CAD build for the part. Positions are in the model's coordinates, mm. A direction names the side the tool comes from. Round coordinates to 2 decimals unless told otherwise and drop trailing zeros. Loops run counter-clockwise (first coordinate to the right, second up) from the corner with the lowest first, then second, coordinate; pieces in that order, holes last.
```python
from build123d import *

# Parameters (mm, degrees)
SKETCH1_W           = 24
SKETCH1_H           = 24
BOSS_EXTRUDE1_DEPTH = 20
SKETCH5_W           = 5
SKETCH5_H           = 4
SKETCH3_W           = 20
SKETCH3_H           = 20
CUT_EXTRUDE5_DEPTH  = 6
SKETCH14_W          = 20
SKETCH14_H          = 20
CUT_EXTRUDE6_DEPTH  = 2
SKETCH15_W          = 17.5
SKETCH15_H          = 17.5
CUT_EXTRUDE7_DEPTH  = 9
CUT_EXTRUDE8_REACH  = 5
SKETCH16_R          = 4.25
CUT_EXTRUDE9_REACH  = 5.25
SKETCH17_R          = 4.25


with BuildPart() as part:
    # Sketch1 → Boss-Extrude1 (new body)
    with BuildSketch(Plane(origin=(0, 0, 0), x_dir=(1, 0, 0), z_dir=(0, 1, 0))):
        Rectangle(SKETCH1_W, SKETCH1_H)
    extrude(amount=BOSS_EXTRUDE1_DEPTH)

    # Sweep1: sweep along a path in Sketch6
    with BuildLine(Plane(origin=(0, 0, 0), x_dir=(0, 0, -1), z_dir=(1, 0, 0))) as sweep1_path:
        Line((12, 16), (15, 16))
        ThreePointArc((15, 16), (17.025627927, 16.352272006), (18.813398517, 17.367722833))
    # Sketch5 → Sweep1 (sweep)
    with BuildSketch(Plane(origin=(0, 0, -12), x_dir=(-1, 0, 0), z_dir=(0, 0, -1))):
        with Locations((0, 16)):
            Rectangle(SKETCH5_W, SKETCH5_H)
    sweep1 = sweep(path=sweep1_path.line)

    # Mirror1: Sweep1 across plane
    add(sweep1.mirror(Plane.XY))

    # Sketch3 → Cut-Extrude5 (cut)
    with BuildSketch(Plane.XZ):
        Rectangle(SKETCH3_W, SKETCH3_H)
    extrude(amount=-CUT_EXTRUDE5_DEPTH, mode=Mode.SUBTRACT)

    # Sketch14 → Cut-Extrude6 (cut)
    with BuildSketch(Plane.XZ.offset(-6)):
        Rectangle(SKETCH14_W, SKETCH14_H)
    extrude(amount=-CUT_EXTRUDE6_DEPTH, mode=Mode.SUBTRACT)

    # Sketch15 → Cut-Extrude7 (cut)
    with BuildSketch(Plane.XZ.offset(-8)):
        Rectangle(SKETCH15_W, SKETCH15_H)
    extrude(amount=-CUT_EXTRUDE7_DEPTH, mode=Mode.SUBTRACT)

    # Sketch16 → Cut-Extrude8 (cut, up to next)
    with BuildSketch(Plane.XZ.offset(-17), mode=Mode.PRIVATE) as cut_extrude8_sk1:
        Circle(SKETCH16_R)
    cut_extrude8_tool1 = extrude(cut_extrude8_sk1.sketch, amount=-CUT_EXTRUDE8_REACH, mode=Mode.PRIVATE) & part.part
    add(cut_extrude8_tool1.solids().sort_by_distance((0, 17, 0))[0], mode=Mode.SUBTRACT)

    # Sketch17 → Cut-Extrude9 (cut, up to next)
    with BuildSketch(Plane.ZY.offset(-8.75), mode=Mode.PRIVATE) as cut_extrude9_sk1:
        with Locations((0, 12.5)):
            Circle(SKETCH17_R)
    cut_extrude9_tool1 = extrude(cut_extrude9_sk1.sketch, amount=-CUT_EXTRUDE9_REACH, mode=Mode.PRIVATE) & part.part
    add(cut_extrude9_tool1.solids().sort_by_distance((8.75, 12.5, 0))[0], mode=Mode.SUBTRACT)


solid = part.part
```
Item 1: Cut at A-A, the plane x = 0. Give the cut face in (y, z).
Answers follow:
outline: (0, -12) - (14, -12) - (14, -15) arc R8 ccw to (15.82, -20.08) - (18.91, -17.54) arc R4 cw to (18, -15) - (18, -12) - (20, -12) - (20, -4.25) - (17, -4.25) - (17, -8.75) - (8, -8.75) - (8, -10) - (0, -10) - close; (0, 10) - (8, 10) - (8, 8.75) - (17, 8.75) - (17, 4.25) - (20, 4.25) - (20, 12) - (18, 12) - (18, 15) arc R4 cw to (18.91, 17.54) - (15.82, 20.08) arc R8 ccw to (14, 15) - (14, 12) - (0, 12) - close
Item 2: Flat gauge pins, fed straight in: P1, Ø5.5, axis at y = 15.5, z = 18, coming from the +X side; P2, Ø3, axis at y = 13, z = 2.5, coming from the +X side; P3, Ø2.5, axis at x = 0, z = 14, coming from the -Y side; P4, Ø6, axis at x = 8.5, z = 11.5, coming from the -Y side. Where does each tip first touch, or does it go through?
Answers follow:
P1: stops at x = 2.5
P2: stops at x = -8.75
P3: stops at y = 14
P4: stops at y = 0
Item 3: Cut at D-D, the plane z = -9.5. Give the cut face in (x, y).
Answers follow:
outline: (-12, 0) - (-10, 0) - (-10, 8) - (10, 8) - (10, 0) - (12, 0) - (12, 20) - (-12, 20) - close
Item 4: 3-axis set-ups, long thin cutter, end or side, ignore diameter. For faces 1 (the flat face through (-10, 4, 0)), 2 (the flat face through (-12, 10, 0)), 3 (the flat face through (2.5, 16, -15)), 4 (the flat face through (0, 18, -14)), 5 (the flat face through (10.5, 0, -0.2)): which of +Z, -Z, +X, -X, +Y, -Y reach the whole face in a straight line?
Answers follow:
face 1: -Y
face 2: +Z, -Z, -X, +Y, -Y
face 3: -Z, +X, +Y, -Y
face 4: +X, -X, +Y
face 5: +Z, -Z, +X, -X, -Y
Item 5: Two-plate mould, pull along Z, no slides. Class faces 6 (the cylindrical face through (-0.035, 14.457, 17.665)), 7 (the cylindrical face through (0.035, 18.228, 16.332)), 8 (the flat face through (-2.5, 16, -15)): released by +Z, released by -Z, zero draft, split by the parting line, or undercut.
Answers follow:
face 6: released by +Z
face 7: undercut
face 8: zero draft
Item 6: Probe line 1 (Z direction, x = 3.5, y = 10); line 2 (Z direction, x = 0.25, y = 6.5). List the from-to ranges inside material, lowest first.
Answers follow:
line 1: z = -12 to -8.75, 8.75 to 12
line 2: z = -12 to -10, 10 to 12
Item 7: Cut at C-C, the plane y = 3.5. Give the cut face in (x, z).
Answers follow:
outline: (-12, -12) - (12, -12) - (12, 12) - (-12, 12) - close; hole (-10, -10) - (10, -10) - (10, 10) - (-10, 10) - close
Item 8: Cut at B-B, the plane z = 0. Give the cut face in (x, y), plus the area to 3 significant figures.
Answers follow:
outline: (-12, 0) - (-10, 0) - (-10, 8) - (-8.75, 8) - (-8.75, 17) - (-4.25, 17) - (-4.25, 20) - (-12, 20) - close; (4.25, 17) - (8.75, 17) - (8.75, 16.75) - (12, 16.75) - (12, 20) - (4.25, 20) - close; (8.75, 8) - (10, 8) - (10, 0) - (12, 0) - (12, 8.25) - (8.75, 8.25) - close
area: 109 mm2
